```python
from build123d import *

# Parameters (mm, degrees)
SKETCH_1_R               = 5
SKETCH_1_R_2             = 2.5
EXTRUDE_1_DEPTH          = 3
SKETCH_2_R               = 5
EXTRUDE_2_DEPTH          = 2
EXTRUDE_3_DEPTH          = 5
SKETCH_6_R               = 1
CUT_EXTRUDE_2_DEPTH      = 10
SKETCH_7_W               = 6
SKETCH_7_H               = 10
EXTRUDE_5_DEPTH          = 10.5
SKETCH_8_R               = 1
CUT_EXTRUDE_3_DEPTH      = 12
CUT_EXTRUDE_4_DEPTH      = 24.135470603
CUT_EXTRUDE_4_DEPTH_BACK = 24.135470603


with BuildPart() as part:
    # 草图1 → 凸台-拉伸1 (new body)
    with BuildSketch(Plane.XY):
        Circle(SKETCH_1_R)
        Circle(SKETCH_1_R_2, mode=Mode.SUBTRACT)
    extrude(amount=EXTRUDE_1_DEPTH)

    # 草图2 → 凸台-拉伸2 (add)
    with BuildSketch(Plane.XY.offset(3)):
        Circle(SKETCH_2_R)
    extrude(amount=EXTRUDE_2_DEPTH)

    # 草图3 → 凸台-拉伸3 (add)
    with BuildSketch(Plane(origin=(0, 0, 0), x_dir=(-1, 0, 0), z_dir=(0, 0, -1))):
        with BuildLine():
            Line((0, 5), (20, 5))
            Line((20, 5), (20, -5))
            Line((20, -5), (0, -5))
            ThreePointArc((0, -5), (5, 0), (0, 5))
        make_face()
    extrude(amount=-EXTRUDE_3_DEPTH)

    # 草图6 → 切除-拉伸2 (cut)
    with BuildSketch(Plane(origin=(0, 5, 0), x_dir=(1, 0, 0), z_dir=(0, 1, 0))):
        with Locations(Location((-17, -2.5, 0), (0, 0, 270))):
            Circle(SKETCH_6_R)
    extrude(amount=-CUT_EXTRUDE_2_DEPTH, mode=Mode.SUBTRACT)

    # 草图7 → 凸台-拉伸5 (add)
    with BuildSketch(Plane(origin=(0, 0, 0), x_dir=(-1, 0, 0), z_dir=(0, 0, -1))):
        with Locations((17, 0)):
            Rectangle(SKETCH_7_W, SKETCH_7_H)
    extrude(amount=EXTRUDE_5_DEPTH)

    # 草图8 → 切除-拉伸3 (cut)
    with BuildSketch(Plane(origin=(0, 5, 0), x_dir=(1, 0, 0), z_dir=(0, 1, 0))):
        with Locations(Location((-17, 7.5, 0), (0, 0, 270))):
            Circle(SKETCH_8_R)
    extrude(amount=-CUT_EXTRUDE_3_DEPTH, mode=Mode.SUBTRACT)

    # 草图9 → 切除-拉伸4 (cut, two sides: drawn at the far end of the back side and taken through both)
    with BuildSketch(Plane(origin=(0, 0, 0), x_dir=(-1, 0, 0), z_dir=(0, 0, -1)).offset(-CUT_EXTRUDE_4_DEPTH_BACK)):
        with BuildLine():
            Line((5, 0), (20, 0))
            Line((20, 0), (20, -5))
            Line((20, -5), (0, -5))
            ThreePointArc((0, -5), (3.535533906, -3.535533906), (5, 0))
        make_face()
    extrude(amount=CUT_EXTRUDE_4_DEPTH + CUT_EXTRUDE_4_DEPTH_BACK, mode=Mode.SUBTRACT)


solid = part.part
```
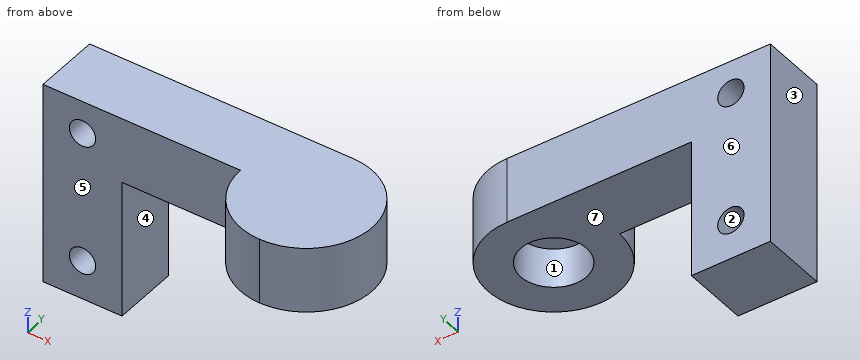
Can you work these out from the model? Positions are in its coordinate system, mm. Face numbers are marked on the shaded views. A direction names the side the tool comes from. Round coordinates to 2 decimals unless told otherwise and drop trailing zeros. Order: outer loops, then holes, each group sorted by start corner. A loop starts at its lowest first (then second) coordinate and runs counter-clockwise, first axis right, second up. Notation, with made-up numbers: (-12, 68) -> (46, 68) arc R10 ccw to (46, 79) -> close; hole circle Ø5 at (72, 89). An arc over 180 degrees is marked (long way). Return JSON: item names as keys, results as strings. Group by question number.
1. I need wall thicknesses on line 1 (X direction, y = 3.8, z = -7.5); line 2 (Z direction, x = -17.75, y = 2.75); line 3 (Y direction, x = 0, z = 0.85). Which ranges of each line are inside material? Lowest first, please. Write a range as [from, to].
2. If we section it at A-A, the plane z = -7.5: Write out the boundary of the cut face in (x, y).
3. We'd pull the mould along X, two halves only. Please class the marked faces 1, 2, 3 and 4: released by +X, released by -X, zero draft, split by the parting line, or undercut.
4. If we section it at B-B, the plane y = 1: Write out the boundary of the cut face in (x, z), then the cut area to 3 significant figures.
5. If we section it at C-C, the plane z = 3.75: Write out the boundary of the cut face in (x, y), then the cut area to 3 significant figures.
6. Will these pins go through, and if not, where does the flat tip stop? pin 1 (8 mm diameter, centred on x = -17.5, z = 2.5, fed in from -Y); pin 2 (3 mm diameter, centred on x = -17, z = -7.5, fed in from +Y); pin 3 (2.5 mm diameter, centred on y = 3.5, z = -3, fed in from +X); pin 4 (3 mm diameter, centred on x = 1, y = -3, fed in from -Z).
7. Which directions (+Z, -Z, +X, -X, +Y, -Y) give clear straight access to the entire face, cutting with the end or side of a thin tool? Please do the marked faces 5, 6 and 7.
8. If we section it at D-D, the plane x = -0.5: Write out the boundary of the cut face in (y, z), then the cut area to 3 significant figures.
Output values:
{
 "1": {"line 1": "[-20, -18], [-16, -14]", "line 2": "[-10.5, -8.16], [-6.84, 1.84], [3.16, 5]", "line 3": "[-5, -2.5], [2.5, 5]"},
 "2": {"outline": "(-20, 0) -> (-18, 0) -> (-18, 5) -> (-20, 5) -> close; (-16, 0) -> (-14, 0) -> (-14, 5) -> (-16, 5) -> close"},
 "3": {"face 1": "undercut", "face 2": "undercut", "face 3": "released by -X", "face 4": "released by +X"},
 "4": {"outline": "(-20, -10.5) -> (-14, -10.5) -> (-14, 0) -> (-2.29, 0) -> (-2.29, 3) -> (2.29, 3) -> (2.29, 0) -> (4.9, 0) -> (4.9, 5) -> (-20, 5) -> close; hole circle Ø2 at (-17, -7.5); hole circle Ø2 at (-17, 2.5)", "area": "167 mm²"},
 "5": {"outline": "(-20, 0) -> (-5, 0) arc R5 ccw (long way) to (0, 5) -> (-20, 5) -> close", "area": "159 mm²"},
 "6": {"pin 1": "y = 0", "pin 2": "y = 5", "pin 3": "x = -14", "pin 4": "z = 0"},
 "7": {"face 5": "+Z, -Z, -X, -Y", "face 6": "+Z, -Z, +X, -X, +Y", "face 7": "-Z, +X, +Y, -Y"},
 "8": {"outline": "(-4.97, 0) -> (-2.45, 0) -> (-2.45, 3) -> (2.45, 3) -> (2.45, 0) -> (5, 0) -> (5, 5) -> (-4.97, 5) -> close", "area": "35.2 mm²"}
}
